Could you check a few things on this model? Use its own coordinates, in mm. Face numbers are marked on the shaded views. Give positions to 0.01 mm unless a question says otherwise; leave off trailing zeros. Write each loop counter-clockwise with the first axis right and the second up, starting at its lowest first coordinate (ties: lowest second). Pieces come first, ordered by that corner, then holes. Notation, with made-up numbers: M -39.75,53.5 L -10.75,53.5 A18 cw -10.75,59.5 Z; hole C 86,77 d11. An arc over 180 degrees is marked long. Write each question's results on one line, items separated by ' | '. Start each with the question number.
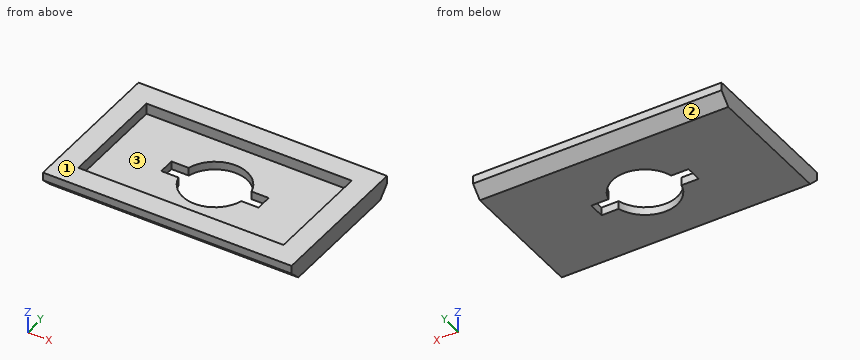
from build123d import *

# Parameters (mm, degrees)
SKETCH_1_W          = 46
SKETCH_1_H          = 28
EXTRUDE_1_DEPTH     = 3.5
SKETCH_2_W          = 38
SKETCH_2_H          = 20
CUT_EXTRUDE_1_DEPTH = 2
CHAMFER_1_SIZE      = 2


with BuildPart() as part:
    # 草图1 → 凸台-拉伸1 (new body)
    with BuildSketch(Plane.XY):
        Rectangle(SKETCH_1_W, SKETCH_1_H)
        with BuildLine():
            Line((5.809475019, 1.5), (9, 1.5))
            Line((9, 1.5), (9, -1.5))
            Line((9, -1.5), (5.809475019, -1.5))
            ThreePointArc((5.809475019, -1.5), (0, -6), (-5.809475019, -1.5))
            Line((-5.809475019, -1.5), (-9, -1.5))
            Line((-9, -1.5), (-9, 1.5))
            Line((-9, 1.5), (-5.809475019, 1.5))
            ThreePointArc((-5.809475019, 1.5), (0, 6), (5.809475019, 1.5))
        make_face(mode=Mode.SUBTRACT)
    extrude(amount=EXTRUDE_1_DEPTH)

    # 草图2 → 切除-拉伸1 (cut)
    with BuildSketch(Plane.XY.offset(3.5)):
        Rectangle(SKETCH_2_W, SKETCH_2_H)
    extrude(amount=-CUT_EXTRUDE_1_DEPTH, mode=Mode.SUBTRACT)

    # 倒角1
    chamfer_1_edges = [part.edges().sort_by_distance(p)[0] for p in [
        (0, -14, 0),
        (0, 14, 0),
    ]]
    chamfer(chamfer_1_edges, length=CHAMFER_1_SIZE)


solid = part.part
Q1. If we section it at D-D (z = 2.9): Please give me the cut outline in (x, y), plus the area to 3 significant figures.
Q2. If we section it at C-C (y = 9.25): Please give me the cut outline in (x, z), plus the area to 3 significant figures.
Q3. I'm going to push flat-ended pins straight in: P1, Ø0.8, axis at x = 8, z = 0.5, coming from the -Y side; P2, Ø1.2, axis at x = 8, z = 1, coming from the +Y side; P3, Ø8, axis at x = 2, y = 5, coming from the +Z side. Where does each tip first touch, or does it pass through?
Q4. If we mould it in two halves opening along Y, with no side actions, what happens to the marked faces 1, 2 and 3? For each: pulls with the +Y half, pulls with the -Y half, needs draft (parallel to the pull), parting line crosses it, or undercut.
Q5. If we section it at A-A (z = 0.7): Please give me the cut outline in (x, y).
Q6. Please list where these lines run through material, in increasing order: line 1 (X direction, y = 8.25, z = 2.15); line 2 (Y direction, x = 17.5, z = 2.95); line 3 (Y direction, x = -5, z = 0.8). Write a range as [from, to].
Q7. If we section it at B-B (x = 7.5): Please give me the cut outline in (y, z).
Determined:
1) outline: M -23,-14 L 23,-14 L 23,14 L -23,14 Z; hole M -19,-10 L 19,-10 L 19,10 L -19,10 Z | area: 528 mm²
2) outline: M -23,0 L 23,0 L 23,3.5 L 19,3.5 L 19,1.5 L -19,1.5 L -19,3.5 L -23,3.5 Z | area: 85.0 mm²
3) P1: stops at y = -12.9 | P2: stops at y = 13.6 | P3: stops at z = 1.5
4) face 1: needs draft | face 2: pulls with the +Y half | face 3: undercut
5) outline: M -23,-12.7 L 23,-12.7 L 23,12.7 L -23,12.7 Z; hole M -9,-1.5 L -5.81,-1.5 A6 ccw 5.81,-1.5 L 9,-1.5 L 9,1.5 L 5.81,1.5 A6 ccw -5.81,1.5 L -9,1.5 Z
6) line 1: x = [-23, -19], [19, 23] | line 2: y = [-14, -10], [10, 14] | line 3: y = [-12.8, -3.32], [3.32, 12.8]
7) outline: M -14,2 L -12,0 L -1.5,0 L -1.5,1.5 L -10,1.5 L -10,3.5 L -14,3.5 Z; M 1.5,0 L 12,0 L 14,2 L 14,3.5 L 10,3.5 L 10,1.5 L 1.5,1.5 Z
